For this review, take the finished solid that the model builds, in its own axes (mm). A direction names the side the tool comes from. Coordinates: 2 decimals unless noted, no trailing zeros. Write each loop counter-clockwise with the first axis right and the second up, starting at its lowest first coordinate (ties: lowest second). Pieces come first, ordered by that corner, then holes. Notation, with made-up numbers: M 49.25,14.25 L 73.25,14.25 A19 ccw 73.25,24.25 Z; hole C 64,17 d5. An arc over 180 degrees is marked long. One line per question, with ' | ' between items.
from build123d import *

# Parameters (mm, degrees)
EXTRUDE_1_DEPTH     = 65
SKETCH_3_W          = 1
SKETCH_3_H          = 14
CUT_EXTRUDE_1_DEPTH = 20
SKETCH_5_W          = 14
SKETCH_5_H          = 1
EXTRUDE_4_DEPTH     = 16
SKETCH_6_W          = 15
SKETCH_6_H          = 1
CUT_EXTRUDE_2_DEPTH = 19
SKETCH_7_W          = 15
SKETCH_7_H          = 1
CUT_EXTRUDE_3_DEPTH = 1


with BuildPart() as part:
    # Эскиз1 → Бобышка-Вытянуть1 (new body)
    with BuildSketch(Plane(origin=(0, 0, 0), x_dir=(1, 0, 0), z_dir=(0, 1, 0))):
        Polygon((0, 0), (0, 15), (1, 15), (1, 1), (15, 1), (15, 0), align=None)
    extrude(amount=EXTRUDE_1_DEPTH)

    # Эскиз3 → Вырез-Вытянуть1 (cut)
    with BuildSketch(Plane.XZ):
        with Locations((0.5, -8)):
            Rectangle(SKETCH_3_W, SKETCH_3_H)
    extrude(amount=-CUT_EXTRUDE_1_DEPTH, mode=Mode.SUBTRACT)

    # Эскиз5 → Бобышка-Вытянуть4 (add)
    with BuildSketch(Plane(origin=(1, 0, 0), x_dir=(0, 0, -1), z_dir=(1, 0, 0))):
        with Locations((8, 19.5)):
            Rectangle(SKETCH_5_W, SKETCH_5_H)
    extrude(amount=-EXTRUDE_4_DEPTH)

    # Эскиз6 → Вырез-Вытянуть2 (cut)
    with BuildSketch(Plane.XZ):
        with Locations((7.5, -0.5)):
            Rectangle(SKETCH_6_W, SKETCH_6_H)
    extrude(amount=-CUT_EXTRUDE_2_DEPTH, mode=Mode.SUBTRACT)

    # Эскиз7 → Вырез-Вытянуть3 (cut)
    with BuildSketch(Plane.XZ.offset(-19)):
        with Locations((7.5, -0.5)):
            Rectangle(SKETCH_7_W, SKETCH_7_H)
    extrude(amount=-CUT_EXTRUDE_3_DEPTH, mode=Mode.SUBTRACT)


solid = part.part
1. Machinability: for faces 1 (the flat face through (0, 42, -7)), 2 (the flat face through (1, 42, -8)), 3 (the flat face through (-15, 19.5, -7.9)), which of the approach directions +Z, -Z, +X, -X, +Y, -Y give a long, thin tool a straight path to every point of the face, cutting with its end or side? Answer none if there is none.
Computed values:
face 1: +Z, -Z, -X, +Y | face 2: -Z, +X, +Y, -Y | face 3: +Z, -Z, -X, +Y, -Y
2. Take a section at D-D on x = -2.25. State the section outline as (y, z) points.
Computed values:
outline: M 19,-15 L 20,-15 L 20,-1 L 19,-1 Z
3. Take a section at A-A on y = 49. State the section outline as (x, z) points, plus the area to 3 significant figures.
Computed values:
outline: M 0,-15 L 1,-15 L 1,-1 L 15,-1 L 15,0 L 0,0 Z | area: 29.0 mm2
4. Take a section at B-B on z = -2. State the section outline as (x, y) points.
Computed values:
outline: M -15,19 L 1,19 L 1,65 L 0,65 L 0,20 L -15,20 Z
5. Take a section at C-C on x = 2.75. State the section outline as (y, z) points, plus the area to 3 significant figures.
Computed values:
outline: M 20,-1 L 65,-1 L 65,0 L 20,0 Z | area: 45.0 mm2
6. For line 1 along Z through (x, y) = (3.25, 41.5); line 2 along Y through (x, z) = (2, -0.5); line 3 along X through (y, z) = (45, -12.25), list the stretches that pass through material, from the lowest coordinate up.
Computed values:
line 1: z = -1 to 0 | line 2: y = 20 to 65 | line 3: x = 0 to 1
7. Clearance check with flat-ended pins moving along their axes: P1, Ø3, axis at y = 26, z = -3, coming from the +X side; P2, Ø0.8, axis at x = 7.5, z = -0.5, coming from the -Y side; P3, Ø7.5, axis at y = 38.5, z = -9, coming from the -X side. State where each tip first meets the part, or that it passes through.
Computed values:
P1: stops at x = 1 | P2: stops at y = 20 | P3: stops at x = 0
